```python
from build123d import *

# Parameters (mm, degrees)
SKETCH1_W           = 108.6
SKETCH1_H           = 58
BOSS_EXTRUDE1_DEPTH = 2.5
SKETCH2_W           = 10
SKETCH2_H           = 58
BOSS_EXTRUDE2_DEPTH = 8.5
SKETCH3_W           = 6
SKETCH3_H           = 58
BOSS_EXTRUDE3_DEPTH = 5
SKETCH4_W           = 6
SKETCH4_H           = 58
BOSS_EXTRUDE4_DEPTH = 5
SKETCH5_W           = 10
SKETCH5_H           = 58
BOSS_EXTRUDE5_DEPTH = 8.5
SKETCH6_W           = 6
SKETCH6_H           = 58
BOSS_EXTRUDE6_DEPTH = 5
SKETCH7_W           = 6
SKETCH7_H           = 58
BOSS_EXTRUDE7_DEPTH = 5
SKETCH8_W           = 108.6
SKETCH8_H           = 22.5
BOSS_EXTRUDE8_DEPTH = 3.5
SKETCH9_R           = 3.15
CUT_EXTRUDE1_DEPTH  = 2.7
SKETCH10_W          = 7
SKETCH10_H          = 3
SKETCH10_W_2        = 7.05
CUT_EXTRUDE2_DEPTH  = 58


with BuildPart() as part:
    # Sketch1 → Boss-Extrude1 (new body)
    with BuildSketch(Plane.XY):
        Rectangle(SKETCH1_W, SKETCH1_H)
    extrude(amount=BOSS_EXTRUDE1_DEPTH)

    # Sketch2 → Boss-Extrude2 (add)
    with BuildSketch(Plane.XY.offset(2.5)):
        with Locations((-37.3, 0)):
            Rectangle(SKETCH2_W, SKETCH2_H)
        with Locations((37.3, 0)):
            Rectangle(SKETCH2_W, SKETCH2_H)
    extrude(amount=BOSS_EXTRUDE2_DEPTH)

    # Sketch3 → Boss-Extrude3 (add)
    with BuildSketch(Plane(origin=(42.3, 0, 0), x_dir=(0, 0, -1), z_dir=(1, 0, 0))):
        with Locations((-8, 0)):
            Rectangle(SKETCH3_W, SKETCH3_H)
    extrude(amount=BOSS_EXTRUDE3_DEPTH)

    # Sketch4 → Boss-Extrude4 (add)
    with BuildSketch(Plane.ZY.offset(42.3)):
        with Locations((8, 0)):
            Rectangle(SKETCH4_W, SKETCH4_H)
    extrude(amount=BOSS_EXTRUDE4_DEPTH)

    # Sketch5 → Boss-Extrude5 (add)
    with BuildSketch(Plane(origin=(0, 0, 0), x_dir=(-1, 0, 0), z_dir=(0, 0, -1))):
        with Locations((-25.7, 0)):
            Rectangle(SKETCH5_W, SKETCH5_H)
        with Locations((25.7, 0)):
            Rectangle(SKETCH5_W, SKETCH5_H)
    extrude(amount=BOSS_EXTRUDE5_DEPTH)

    # Sketch6 → Boss-Extrude6 (add)
    with BuildSketch(Plane(origin=(30.7, 0, 0), x_dir=(0, 0, -1), z_dir=(1, 0, 0))):
        with Locations((5.5, 0)):
            Rectangle(SKETCH6_W, SKETCH6_H)
    extrude(amount=BOSS_EXTRUDE6_DEPTH)

    # Sketch7 → Boss-Extrude7 (add)
    with BuildSketch(Plane.ZY.offset(30.7)):
        with Locations((-5.5, 0)):
            Rectangle(SKETCH7_W, SKETCH7_H)
    extrude(amount=BOSS_EXTRUDE7_DEPTH)

    # Sketch8 → Boss-Extrude8 (add)
    with BuildSketch(Plane.XZ.offset(29)):
        with Locations((0, 1.25)):
            Rectangle(SKETCH8_W, SKETCH8_H)
    extrude(amount=BOSS_EXTRUDE8_DEPTH)

    # Sketch9 → Cut-Extrude1 (cut)
    with BuildSketch(Plane(origin=(0, -29, 0), x_dir=(1, 0, 0), z_dir=(0, 1, 0))):
        with Locations(Location((-39.45, 5.625, 0), (0, 0, 270))):
            Circle(SKETCH9_R)
        with Locations(Location((-50.925, -8.125, 0), (0, 0, 270))):
            Circle(SKETCH9_R)
        with Locations(Location((39.45, 5.625, 0), (0, 0, 270))):
            Circle(SKETCH9_R)
        with Locations(Location((50.925, -8.125, 0), (0, 0, 270))):
            Circle(SKETCH9_R)
    extrude(amount=-CUT_EXTRUDE1_DEPTH, mode=Mode.SUBTRACT)

    # Sketch10 → Cut-Extrude2 (cut)
    with BuildSketch(Plane(origin=(0, 29, 0), x_dir=(1, 0, 0), z_dir=(0, 1, 0))):
        with Locations((28.95, 7)):
            Rectangle(SKETCH10_W, SKETCH10_H)
        with Locations((-29.05, 7)):
            Rectangle(SKETCH10_W, SKETCH10_H)
        with Locations((-39.3, -9.5)):
            Rectangle(SKETCH10_W, SKETCH10_H)
        with Locations((35.805, -9.5)):
            Rectangle(SKETCH10_W_2, SKETCH10_H)
    extrude(amount=-CUT_EXTRUDE2_DEPTH, mode=Mode.SUBTRACT)


solid = part.part
```
Can you work these out from the model? Positions are in its coordinate system, mm. A direction names the side the tool comes from. Coordinates: 2 decimals unless noted, no trailing zeros. Loops run counter-clockwise (first coordinate to the right, second up) from the corner with the lowest first, then second, coordinate; pieces in that order, holes last. Notation, with made-up numbers: (-33, 82) - (-6, 82) arc R26 ccw to (-6, 107) - close; hole circle Ø11 at (-23.5, -4.5). An arc over 180 degrees is marked (long way). Use a Markdown table: item, result.
Item 1: We'd pull the mould along X, two halves only. Please class faces 4 (the face through (-35.7, 0, -6)), 5 (the face through (42.573, -30.331, -6.035)), 6 (the face through (35.7, 0, -5)): released by +X, released by -X, zero draft, split by the parting line, or undercut.
Numbers:
| item | result |
|---|---|
| face 4 | released by -X |
| face 5 | undercut |
| face 6 | released by +X |
Item 2: For faces 1 (the face through (-42.3, 0, 4)), 2 (the face through (36, 0, 8)), 3 (the face through (48, 0, 2.5)), which set-ups out of +Z, -Z, +X, -X, +Y, -Y let a thin tool reach every point of the face, with its end or its side?
Numbers:
| item | result |
|---|---|
| face 1 | -X, +Y |
| face 2 | +Z, +Y |
| face 3 | +X, +Y |
Item 3: I want a section at A-A on x = 34.5. Please give me the cut outline in (y, z), and give its area (3 significant figures).
Numbers:
| item | result |
|---|---|
| outline | (-32.5, -10) - (-29, -10) - (-29, -8.5) - (29, -8.5) - (29, -2.5) - (-29, -2.5) - (-29, 0) - (29, 0) - (29, 8) - (-29, 8) - (-29, 12.5) - (-32.5, 12.5) - close |
| area | 891 mm2 |
Item 4: Will these pins go through, and if not, where does the flat tip stop? pin 1 (1.9 mm diameter, centred on x = 39, z = -6.5, fed in from +Y); pin 2 (10 mm diameter, centred on x = 22, y = 2.5, fed in from -Z); pin 3 (3.5 mm diameter, centred on x = -39.5, y = 5, fed in from +Z).
Numbers:
| item | result |
|---|---|
| pin 1 | stops at y = -31.7 |
| pin 2 | stops at z = -8.5 |
| pin 3 | stops at z = 8 |
Item 5: I want a section at D-D on x = -8. Please give me the cut outline in (y, z), and give its area (3 significant figures).
Numbers:
| item | result |
|---|---|
| outline | (-32.5, -10) - (-29, -10) - (-29, 0) - (29, 0) - (29, 2.5) - (-29, 2.5) - (-29, 12.5) - (-32.5, 12.5) - close |
| area | 224 mm2 |
Item 6: I want a section at C-C on x = -39.45. Please give me the cut outline in (y, z) (3 decimals).
Numbers:
| item | result |
|---|---|
| outline | (-32.5, -10) - (-29, -10) - (-29, -8.775) - (-31.7, -8.775) - (-31.7, -2.475) - (-29, -2.475) - (-29, 0) - (29, 0) - (29, 8) - (-29, 8) - (-29, 12.5) - (-32.5, 12.5) - close |
Item 7: If I drill on probe 1 along X at (y, z) = (-3.5, 9); probe 2 along X at (y, z) = (-20, -8.25); probe 3 along X at (y, z) = (24, -4), over which ranges is the centre line in solid material (lowest first)? Write a range as from..to.
Numbers:
| item | result |
|---|---|
| probe 1 | x = -47.3..-42.8, -35.8..-32.3, 39.33..47.3 |
| probe 2 | x = -35.7..-32.55, -25.55..-20.7, 20.7..25.45, 32.45..35.7 |
| probe 3 | x = -35.7..-20.7, 20.7..35.7 |
Item 8: I want a section at B-B on z = 6.25. Please give me the cut outline in (x, y).
Numbers:
| item | result |
|---|---|
| outline | (-54.3, -32.5) - (54.3, -32.5) - (54.3, -29) - (53.46, -29) - (53.46, -31.7) - (48.39, -31.7) - (48.39, -29) - (47.3, -29) - (47.3, 29) - (32.3, 29) - (32.3, -29) - (-32.3, -29) - (-32.3, 29) - (-47.3, 29) - (-47.3, -29) - (-48.39, -29) - (-48.39, -31.7) - (-53.46, -31.7) - (-53.46, -29) - (-54.3, -29) - close |
